Geometry check sheet. Reference: the model listing, model coordinates, mm. A direction names the side the tool comes from. Round coordinates to 2 decimals unless told otherwise and drop trailing zeros. Loops run counter-clockwise (first coordinate to the right, second up) from the corner with the lowest first, then second, coordinate; pieces in that order, holes last. Notation, with made-up numbers: (-8, -22) -> (0, -22) arc R5 cw to (0, -13) -> close; hole circle Ø11 at (71.5, 36.5). An arc over 180 degrees is marked (long way). Use a Markdown table: item, result. Add a question column.
Q1. Gauge pin test, flat ends, axial feed: P1, Ø1, axis at y = 1, z = -1.5, coming from the -X side; P2, Ø0.8, axis at y = 1.5, z = 1, coming from the +X side; P3, Ø4, axis at x = 0, z = 0, coming from the +Y side. Record the tip position at first contact, or that the pin passes through.
Q2. Sectioned sample at D-D, the plane z = 4.75. Enter the section's corners in (x, y), then the cut area to 3 significant figures.
Q3. Set-up check for faces 1 (the face through (0, 1, 2.476)), 2 (the face through (0, 0, 0)): record each of +Z, -Z, +X, -X, +Y, -Y from which the full face is reachable in a straight line by a thin tool's end or side.
Q4. Sectioned sample at B-B, the plane x = 0. Enter the section's corners in (y, z).
Q5. Material ranges on L1, parallel to Z at x = -2, y = 1.35; L2, parallel to Y at x = 0.25, z = 2.25, recorded low to high.
Q6. Sectioned sample at A-A, the plane z = 0. Enter the section's corners in (x, y).
Q7. Release check for a two-part mould opening along X. For faces 3 (the face through (-2.476, 1, 0)), 4 (the face through (2.476, 1, 0)), 5 (the face through (0, 1.651, 0)), 6 (the face through (0, 1, -2.476)) record: released by +X, released by -X, zero draft, split by the parting line, or undercut.
Q8. Sectioned sample at C-C, the plane y = 0.6. Enter the section's corners in (x, z), then the cut area to 3 significant figures.
```python
from build123d import *

# Parameters (mm, degrees)
SKETCH1_W           = 6.9088
SKETCH1_H           = 9.9568
BOSS_EXTRUDE1_DEPTH = 0.127
SKETCH3_W           = 4.953
SKETCH3_H           = 4.953
BOSS_EXTRUDE3_DEPTH = 1.651
SKETCH5_R           = 2.348345572
CUT_EXTRUDE1_DEPTH  = 0.127


with BuildPart() as part:
    # Sketch1 → Boss-Extrude1 (new body)
    with BuildSketch(Plane(origin=(0, 0, 0), x_dir=(1, 0, 0), z_dir=(0, 1, 0))):
        Rectangle(SKETCH1_W, SKETCH1_H)
    extrude(amount=BOSS_EXTRUDE1_DEPTH)

    # Sketch3 → Boss-Extrude3 (add)
    with BuildSketch(Plane(origin=(0, 0.127, 0), x_dir=(1, 0, 0), z_dir=(0, 1, 0))):
        Rectangle(SKETCH3_W, SKETCH3_H)
    extrude(amount=BOSS_EXTRUDE3_DEPTH)

    # Sketch5 → Cut-Extrude1 (cut)
    with BuildSketch(Plane(origin=(0, 1.778, 0), x_dir=(1, 0, 0), z_dir=(0, 1, 0))):
        Circle(SKETCH5_R)
    extrude(amount=-CUT_EXTRUDE1_DEPTH, mode=Mode.SUBTRACT)


solid = part.part
```
Values:
| question | item | result |
|---|---|---|
| 1 | P1 | x = -2.48 |
| 1 | P2 | x = 2.48 |
| 1 | P3 | y = 1.65 |
| 2 | outline | (-3.45, 0) -> (3.45, 0) -> (3.45, 0.13) -> (-3.45, 0.13) -> close |
| 2 | area | 0.877 mm^2 |
| 3 | face 1 | +Z, +X, -X, +Y |
| 3 | face 2 | +Z, -Z, +X, -X, -Y |
| 4 | outline | (0, -4.98) -> (0.13, -4.98) -> (0.13, -2.48) -> (1.78, -2.48) -> (1.78, -2.35) -> (1.65, -2.35) -> (1.65, 2.35) -> (1.78, 2.35) -> (1.78, 2.48) -> (0.13, 2.48) -> (0.13, 4.98) -> (0, 4.98) -> close |
| 5 | L1 | -2.48 to 2.48 |
| 5 | L2 | 0 to 1.65 |
| 6 | outline | (-3.45, 0) -> (3.45, 0) -> (3.45, 0.13) -> (2.48, 0.13) -> (2.48, 1.78) -> (2.35, 1.78) -> (2.35, 1.65) -> (-2.35, 1.65) -> (-2.35, 1.78) -> (-2.48, 1.78) -> (-2.48, 0.13) -> (-3.45, 0.13) -> close |
| 7 | face 3 | released by -X |
| 7 | face 4 | released by +X |
| 7 | face 5 | undercut |
| 7 | face 6 | zero draft |
| 8 | outline | (-2.48, -2.48) -> (2.48, -2.48) -> (2.48, 2.48) -> (-2.48, 2.48) -> close |
| 8 | area | 24.5 mm^2 |
